Check sheet for the modelled part. Datum: model origin and axes. Units: mm. A direction names the side the tool comes from. Coordinates: 2 decimals unless noted, no trailing zeros. Order: outer loops, then holes, each group sorted by start corner. A loop starts at its lowest first (then second) coordinate and runs counter-clockwise, first axis right, second up.
from build123d import *

# Parameters (mm, degrees)
F0_W          = 10
F0_H          = 22
F0_W_2        = 22
F0_H_2        = 5.75
F0_W_3        = 1.5
F1_DEPTH      = 0.75
F1_DEPTH_BACK = 0.75
F2_W          = 1.5
F2_H          = 22
F3_DEPTH      = 10
F4_W          = 22
F4_H          = 1.5
F5_DEPTH      = 10
F6_R          = 1
F7_DEPTH      = 32.001
F7_DEPTH_BACK = 1.5
F8_R          = 1
F9_DEPTH      = 1.5


with BuildPart() as f1:
    # F0 (on Top) → F1 (new body, two sides)
    with BuildSketch(Plane.XY) as f1_sk:
        with Locations((-11.75, 0)):
            Rectangle(F0_W, F0_H)
        with Locations((4.25, 13.875)):
            Rectangle(F0_W_2, F0_H_2)
        with Locations((4.25, 0)):
            Rectangle(F0_W_2, F0_H)
        with Locations((16, 0)):
            Rectangle(F0_W_3, F0_H)
        with Locations((4.25, -13.875)):
            Rectangle(F0_W_2, F0_H_2)
    extrude(amount=F1_DEPTH)
    extrude(f1_sk.sketch, amount=-F1_DEPTH_BACK)

    # F2 (on face) → F3 (join)
    with BuildSketch(Plane.XY.offset(0.75)):
        with Locations((-16, 0)):
            Rectangle(F2_W, F2_H)
        with Locations((16, 0)):
            Rectangle(F2_W, F2_H)
    extrude(amount=F3_DEPTH)

    # F4 (on face) → F5 (join)
    with BuildSketch(Plane(origin=(0, 0, -0.75), x_dir=(1, 0, 0), z_dir=(0, 0, -1))):
        with Locations((4.25, 16)):
            Rectangle(F4_W, F4_H)
    extrude(amount=F5_DEPTH)

    # F6 (on face) → F7 (cut, two sides)
    with BuildSketch(Plane.YZ.offset(-15.25)) as f7_sk:
        with Locations((-8, 7.25)):
            Circle(F6_R)
        with Locations((8, 7.25)):
            Circle(F6_R)
    extrude(amount=F7_DEPTH, mode=Mode.SUBTRACT)
    extrude(f7_sk.sketch, amount=-F7_DEPTH_BACK, mode=Mode.SUBTRACT)

    # F8 (on face) → F9 (cut, through all)
    with BuildSketch(Plane.XZ.offset(16.75)):
        with Locations((-3.75, -7.25)):
            Circle(F8_R)
        with Locations((12.25, -7.25)):
            Circle(F8_R)
    extrude(amount=-F9_DEPTH, mode=Mode.SUBTRACT)

    # F10: F1 across plane


with BuildPart() as f1_1:
    add(f1.part)
    add(f1.part.mirror(Plane.XZ))


solid = f1_1.part
(1) Tool access check on faces 4 (the flat face through (-16, 0, 10.75)), 5 (the flat face through (-6.75, -15.4, -3.7)), 6 (the flat face through (4, -15.25, -6)), 7 (the flat face through (-15.25, 0, 6)), 8 (the flat face through (-6.75, 15.4, -3.7)). Record the directions out of +Z, -Z, +X, -X, +Y, -Y that give a thin tool (end or side, any length) a straight path to the whole face; none if there is none.
Filled in:
face 4: +Z, +X, -X, +Y, -Y
face 5: +Z, -Z, -X, -Y
face 6: -Z, +X, -X
face 7: +Z, +Y, -Y
face 8: +Z, -Z, -X, +Y
(2) Cross-section at A-A (x = -3.75). Enter the section's corners in (y, z), and give its area (4 significant figures).
Filled in:
outline: (-16.75, -10.75) - (-15.25, -10.75) - (-15.25, -8.25) - (-16.75, -8.25) - close; (-16.75, -6.25) - (-15.25, -6.25) - (-15.25, -0.75) - (15.25, -0.75) - (15.25, -6.25) - (16.75, -6.25) - (16.75, 0.75) - (-16.75, 0.75) - close; (15.25, -10.75) - (16.75, -10.75) - (16.75, -8.25) - (15.25, -8.25) - close
area: 74.25 mm2
(3) Cross-section at B-B (z = 1.5). Enter the section's corners in (x, y), and give its area (3 significant figures).
Filled in:
outline: (-16.75, -11) - (-15.25, -11) - (-15.25, 11) - (-16.75, 11) - close; (15.25, -11) - (16.75, -11) - (16.75, 11) - (15.25, 11) - close
area: 66.0 mm2
(4) Cross-section at D-D (z = -7.25). Enter the section's corners in (x, y), and give its area (3 significant figures).
Filled in:
outline: (-6.75, -16.75) - (-4.75, -16.75) - (-4.75, -15.25) - (-6.75, -15.25) - close; (-6.75, 15.25) - (-4.75, 15.25) - (-4.75, 16.75) - (-6.75, 16.75) - close; (-2.75, -16.75) - (11.25, -16.75) - (11.25, -15.25) - (-2.75, -15.25) - close; (-2.75, 15.25) - (11.25, 15.25) - (11.25, 16.75) - (-2.75, 16.75) - close; (13.25, -16.75) - (15.25, -16.75) - (15.25, -15.25) - (13.25, -15.25) - close; (13.25, 15.25) - (15.25, 15.25) - (15.25, 16.75) - (13.25, 16.75) - close
area: 54.0 mm2
(5) Cross-section at C-C (y = 8). Enter the section's corners in (x, z).
Filled in:
outline: (-16.75, -0.75) - (16.75, -0.75) - (16.75, 6.25) - (15.25, 6.25) - (15.25, 0.75) - (-15.25, 0.75) - (-15.25, 6.25) - (-16.75, 6.25) - close; (-16.75, 8.25) - (-15.25, 8.25) - (-15.25, 10.75) - (-16.75, 10.75) - close; (15.25, 8.25) - (16.75, 8.25) - (16.75, 10.75) - (15.25, 10.75) - close
(6) Thickness scan on probe 1 along X at (y, z) = (1.5, 3); probe 2 along Z at (x, y) = (-3.75, 16.05). Record the ranges inside material, lowest first.
Filled in:
probe 1: x = -16.75 to -15.25, 15.25 to 16.75
probe 2: z = -10.75 to -8.25, -6.25 to 0.75
(7) Release check for a two-part mould opening along X. For faces 1 (the flat face through (-16.75, 0, 5)), 2 (the flat face through (15.25, 0, 6)), 3 (the cylindrical face through (-15.99, -8.13, 8.24)) record: +X half, -X half, draft (parallel to the pull), parting line (faces both ways), or undercut.
Filled in:
face 1: -X half
face 2: undercut
face 3: draft
(8) Go/stop test with flat-tipped pins: P1, Ø1.7, axis at y = -15, z = -3, coming from the +X side; P2, Ø5, axis at x = -13.5, y = -4.5, coming from the -Z side; P3, Ø3, axis at y = 14, z = -2.5, coming from the -X side. Record where each tip stops, or that it passes through.
Filled in:
P1: stops at x = 15.25
P2: stops at z = -0.75
P3: stops at x = -6.75
